Geometry: final body of the model. Coordinates: model frame, mm. A direction names the side the tool comes from. Give positions to 0.01 mm unless a question says otherwise; leave off trailing zeros. Order: outer loops, then holes, each group sorted by start corner. A loop starts at its lowest first (then second) coordinate and runs counter-clockwise, first axis right, second up. Notation, with made-up numbers: (-38.5, -34) - (-7.5, -34) arc R37 cw to (-7.5, 2) - close; hole circle Ø1 at (-9, -19). An arc over 180 degrees is marked (long way). One line per item, written item: value.
```python
from build123d import *

# Parameters (mm, degrees)
SKETCH1_R           = 7.9
SKETCH2_R           = 6.9
SKETCH4_R           = 4
SKETCH3_R           = 4.9
SKETCH7_W           = 12
SKETCH7_H           = 1.2
BOSS_EXTRUDE2_DEPTH = 3
SKETCH8_R           = 4.970098948
SKETCH8_R_2         = 3.95
BOSS_EXTRUDE3_DEPTH = 2.6
CHAMFER1_SIZE       = 0.436764281
CHAMFER1_SIZE_2     = 1.2


# Read off the part's stored shape, not the designer's step: Shell1
with BuildPart() as part:
    # Sketch1 → Loft1 section 0
    with BuildSketch(Plane(origin=(0, 0, 0), x_dir=(1, 0, 0), z_dir=(0, 1, 0))):
        Circle(SKETCH1_R)
    # Sketch2 → Loft1 section 1
    with BuildSketch(Plane(origin=(0, 8, 0), x_dir=(1, 0, 0), z_dir=(0, 1, 0))):
        Circle(SKETCH2_R)
    loft()

    # Sketch4 → Cut-Loft2 section 0
    with BuildSketch(Plane(origin=(0, 3.8, 0), x_dir=(1, 0, 0), z_dir=(0, 1, 0))):
        Circle(SKETCH4_R)
    # Sketch3 → Cut-Loft2 section 1
    with BuildSketch(Plane(origin=(0, 8, 0), x_dir=(1, 0, 0), z_dir=(0, 1, 0))):
        Circle(SKETCH3_R)
    loft(mode=Mode.SUBTRACT)

    # Sketch7 → Boss-Extrude2 (add)
    with BuildSketch(Plane(origin=(0, 6.8, 0), x_dir=(1, 0, 0), z_dir=(0, 1, 0))):
        Rectangle(SKETCH7_W, SKETCH7_H)
    extrude(amount=-BOSS_EXTRUDE2_DEPTH)

    # Shell1 outline → Shell1 (revolve, cut)
    with BuildSketch(Plane.XY):
        Polygon((5.851506773, 6.713236516), (4.970098948, 2.6), (0, 2.6), (0, 0), (6.690661338, 0), align=None)
    revolve(axis=Axis((0, 0, 0), (0, 1, 0)), mode=Mode.SUBTRACT)

    # Sketch8 → Boss-Extrude3 (add)
    with BuildSketch(Plane.XZ.offset(-2.6)):
        with Locations(Location((0, 0, 0), (0, 0, 90))):
            Circle(SKETCH8_R)
        with Locations(Location((0, 0, 0), (0, 0, 90))):
            Circle(SKETCH8_R_2, mode=Mode.SUBTRACT)
    extrude(amount=BOSS_EXTRUDE3_DEPTH)

    # Chamfer1
    # the kernel refuses this chamfer: 1.2, 0.436764281 mm, written as the material it takes off along each edge
    with BuildSketch(Plane(origin=(0, 0, 0), x_dir=(0, 0, 1), z_dir=(1, 0, 0))) as chamfer1_piece_1:
        Polygon((4.970098948, -CHAMFER1_SIZE), (4.970098948 - CHAMFER1_SIZE_2, 0), (4.970098948, 0), align=None)
    revolve(axis=Axis((0, 0, 0), (0, -1, 0)), mode=Mode.SUBTRACT)


solid = part.part
```
1) Mould query, pull axis Z, two halves, no side actions, for faces 1 (the face through (0, 6.8, 0)), 2 (the face through (-2.67, 1.35, -2.91)), 3 (the face through (-5, 8, 1)), 4 (the face through (6.727, 4.945, 2.789)). Classes: released by +Z, released by -Z, zero draft, split by the parting line, or undercut.
Answers below:
face 1: undercut
face 2: undercut
face 3: zero draft
face 4: split by the parting line
2) Section D-D, the plane y = 6.5. Return loops of the section in (x, z) (1 decimal), then the cut area to 3 significant figures.
Answers below:
outline: circle Ø14.2 at (0, 0); circle Ø11.6 at (0, 0); hole circle Ø11.8 at (0, 0); hole (-4.5, -0.6) arc R4.6 ccw to (4.5, -0.6) - close; hole (-4.5, 0.6) - (4.5, 0.6) arc R4.6 ccw to start
area: 100 mm^2
3) Material intervals for line 1 along X through (y, z) = (1.75, 0.5); line 2 along X through (y, z) = (3, 1.75); line 3 along X through (y, z) = (1.5, 0), sorted ascending.
Answers below:
line 1: -7.66 to -6.45, -4.94 to -3.92, 3.92 to 4.94, 6.45 to 7.66
line 2: -7.32 to -6.07, -4.74 to 4.74, 6.07 to 7.32
line 3: -7.71 to -6.5, -4.97 to -3.95, 3.95 to 4.97, 6.5 to 7.71
4) First-contact query: pin 1 (1.5 mm diameter, centred on x = 0.5, y = 5.5, fed in from -Z); pin 2 (1 mm diameter, centred on x = -0.5, z = 0, fed in from +Y); pin 3 (4 mm diameter, centred on x = 1.5, z = 1, fed in from -Y). Flat tips, straight axial feed; report the tip coordinate or a pass-through.
Answers below:
pin 1: z = -7.3
pin 2: y = 6.8
pin 3: y = 2.6
5) Set-up query: faces 5 (the face through (0, 2.6, 0)), 6 (the face through (-6, 0, -4)), 7 (the face through (0, 5, 0.6)). Return all of +Z, -Z, +X, -X, +Y, -Y with unobstructed straight access to the full face (end or side cutting, diameter ignored); none if empty.
Answers below:
face 5: -Y
face 6: +Z, -Z, +X, -X, -Y
face 7: +Y
6) Section B-B, the plane x = 0. Return loops of the section in (y, z).
Answers below:
outline: (0, -7.9) - (8, -6.9) - (8, -4.9) - (3.8, -4) - (3.8, -0.6) - (6.8, -0.6) - (6.8, 0.6) - (3.8, 0.6) - (3.8, 4) - (8, 4.9) - (8, 6.9) - (0, 7.9) - (0, 6.69) - (6.71, 5.85) - (2.6, 4.97) - (0.44, 4.97) - (0.07, 3.95) - (2.6, 3.95) - (2.6, -3.95) - (0.07, -3.95) - (0.44, -4.97) - (2.6, -4.97) - (6.71, -5.85) - (0, -6.69) - close
7) Section C-C, the plane y = 2. Return loops of the section in (x, z), then the cut area to 3 significant figures.
Answers below:
outline: circle Ø15.3 at (0, 0); circle Ø9.94 at (0, 0); hole circle Ø12.88 at (0, 0); hole circle Ø7.9 at (0, 0)
area: 82.1 mm^2
8) Section A-A, the plane y = 4. Return loops of the section in (x, z).
Answers below:
outline: circle Ø14.8 at (0, 0); circle Ø10.54 at (0, 0); hole circle Ø12.38 at (0, 0); hole (-4, -0.6) arc R4.04 ccw to (4, -0.6) - close; hole (-4, 0.6) - (4, 0.6) arc R4.04 ccw to start
